from build123d import *

# Parameters (mm, degrees)
F1_DEPTH = 6.35
F3_DEPTH = 25.4


with BuildPart() as f1:
    # F0 (on Top) → F1 (new body)
    with BuildSketch(Plane.XY):
        Polygon((32.995568, -57.15), (65.991136, 0), (32.995568, 57.15), (-32.995568, 57.15), (-65.991136, 0), (-32.995568, -57.15), align=None)
    extrude(amount=-F1_DEPTH)

    # F2 (on Top) → F3 (join)
    with BuildSketch(Plane.XY):
        Polygon((31.529098, -54.61), (63.058196, 0), (31.529098, 54.61), (-31.529098, 54.61), (-63.058196, 0), (-31.529098, -54.61), align=None)
        Polygon((29.329394, 50.8), (58.658787, 0), (29.329394, -50.8), (-29.329394, -50.8), (-58.658787, 0), (-29.329394, 50.8), align=None, mode=Mode.SUBTRACT)
    extrude(amount=F3_DEPTH)


solid = f1.part
Build history of the part. All positions in model axes, mm. A direction names the side the tool comes from. Round coordinates to 2 decimals unless told otherwise and drop trailing zeros. Loops run counter-clockwise (first coordinate to the right, second up) from the corner with the lowest first, then second, coordinate; pieces in that order, holes last. Notation, with made-up numbers: (86.25, 87) -> (137.25, 87) arc R9 ccw to (137.25, 92) -> close; hole circle Ø1 at (53.5, 17). An arc over 180 degrees is marked (long way). Answer in a Markdown table with one row per item.
Item 1: Pin check, flat tips, straight feed: pin 1 (6 mm diameter, centred on x = -8.5, z = 9, fed in from +Y); pin 2 (12 mm diameter, centred on x = 10.5, z = 4.5, fed in from +Y); pin 3 (2 mm diameter, centred on y = -33.5, z = 6.5, fed in from +X); pin 4 (10 mm diameter, centred on y = 37, z = 0, fed in from +X). Stop position of each tip, or through.
Answers below:
| item | result |
|---|---|
| pin 1 | stops at y = 54.61 |
| pin 2 | stops at y = 57.15 |
| pin 3 | stops at x = 44.29 |
| pin 4 | stops at x = 47.52 |
Item 2: Saw through at D-D (z = -2). Write the cut outline in (x, y).
Answers below:
| item | result |
|---|---|
| outline | (-65.99, 0) -> (-33, -57.15) -> (33, -57.15) -> (65.99, 0) -> (33, 57.15) -> (-33, 57.15) -> close |
Item 3: Which spindle directions (+Z, -Z, +X, -X, +Y, -Y) get a long thin tool onto all of the face, cutting with end or side? Do faces 1 (the flat face through (-47.07, 27.69, 12.52)), 2 (the flat face through (47.07, -27.69, 12.52)), 3 (the flat face through (0, 50.8, 13)), 4 (the flat face through (0, 54.61, 13)). Say none if no direction does.
Answers below:
| item | result |
|---|---|
| face 1 | +Z, -X, +Y |
| face 2 | +Z, +X, -Y |
| face 3 | +Z |
| face 4 | +Z, +X, -X, +Y |
Item 4: Saw through at B-B (x = 4.5). Write the cut outline in (y, z).
Answers below:
| item | result |
|---|---|
| outline | (-57.15, -6.35) -> (57.15, -6.35) -> (57.15, 0) -> (54.61, 0) -> (54.61, 25.4) -> (50.8, 25.4) -> (50.8, 0) -> (-50.8, 0) -> (-50.8, 25.4) -> (-54.61, 25.4) -> (-54.61, 0) -> (-57.15, 0) -> close |
Item 5: Saw through at A-A (z = 22). Write the cut outline in (x, y), and give its area (3 significant figures).
Answers below:
| item | result |
|---|---|
| outline | (-63.06, 0) -> (-31.53, -54.61) -> (31.53, -54.61) -> (63.06, 0) -> (31.53, 54.61) -> (-31.53, 54.61) -> close; hole (-58.66, 0) -> (-29.33, -50.8) -> (29.33, -50.8) -> (58.66, 0) -> (29.33, 50.8) -> (-29.33, 50.8) -> close |
| area | 1,390 mm² |
Item 6: Saw through at C-C (y = -43.5). Write the cut outline in (x, z), and give its area (3 significant figures).
Answers below:
| item | result |
|---|---|
| outline | (-40.88, -6.35) -> (40.88, -6.35) -> (40.88, 0) -> (37.94, 0) -> (37.94, 25.4) -> (33.54, 25.4) -> (33.54, 0) -> (-33.54, 0) -> (-33.54, 25.4) -> (-37.94, 25.4) -> (-37.94, 0) -> (-40.88, 0) -> close |
| area | 743 mm² |
Item 7: Mould opens along X. For faces 5 (the flat face through (0, 57.15, -3)), 6 (the flat face through (49.26, -28.98, -3.13)), 7 (the flat face through (44.2, -25.04, 12.52)) say: +X half, -X half, draft (parallel to the pull), parting line (faces both ways), or undercut.
Answers below:
| item | result |
|---|---|
| face 5 | draft |
| face 6 | +X half |
| face 7 | undercut |
Item 8: Drill centre lines: L1, parallel to Y at x = 3.5, z = 6; L2, parallel to Z at x = 10, y = 15.5; L3, parallel to Y at x = -49, z = 11. Where is each one in solid material? Low to high. Write a range as [from, to].
Answers below:
| item | result |
|---|---|
| L1 | y = [-54.61, -50.8], [50.8, 54.61] |
| L2 | z = [-6.35, 0] |
| L3 | y = [-24.35, -16.73], [16.73, 24.35] |
